from build123d import *

# Parameters (mm, degrees)
F0_R     = 1.25
F1_DEPTH = 18
F2_R     = 6.35
F3_DEPTH = 59.8157


with BuildPart() as f1:
    # F0 (on Top) → F1 (new body)
    with BuildSketch(Plane.XY):
        with BuildLine():
            ThreePointArc((-20.879116, -13.75), (7.17712, -23.947629), (25, 0))
            ThreePointArc((25, 0), (7.17712, 23.947629), (-20.879116, 13.75))
            Line((-20.879116, 13.75), (-20.879116, -13.75))
        make_face()
        Circle(F0_R, mode=Mode.SUBTRACT)
    extrude(amount=F1_DEPTH)

    # F2 (on face) → F3 (cut)
    with BuildSketch(Plane(origin=(-20.879116, 0, 0), x_dir=(0, -1, 0), z_dir=(-1, 0, 0))):
        with Locations((0, 9)):
            Circle(F2_R)
    extrude(amount=-F3_DEPTH, mode=Mode.SUBTRACT)


solid = f1.part
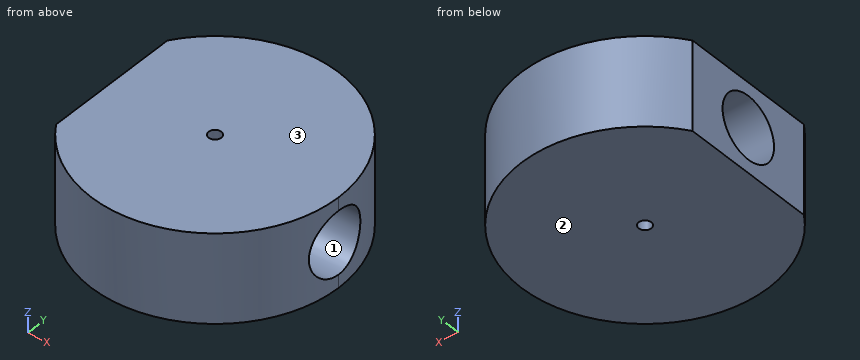
Can you work these out from the model? Positions are in its coordinate system, mm. Face numbers are marked on the shaded views. Give positions to 0.01 mm unless a question says otherwise; leave off trailing zeros. Loops run counter-clockwise (first coordinate to the right, second up) from the corner with the lowest first, then second, coordinate; pieces in that order, holes last. Notation, with made-up numbers: M 75,53.25 L 117,53.25 A27 cw 117,69.25 Z; hole C 72.25,-37 d9. An arc over 180 degrees is marked long. One line per item, written item: value. Start each with the question number.
1) If we section it at C-C, the plane z = 9: Write out the boundary of the cut face in (x, y).
2) If we section it at B-B, the plane y = -3: Write out the boundary of the cut face in (x, z), and give its area (3 significant figures).
3) I'm going to push flat-ended pins straight in: pin 1 (5 mm diameter, centred on x = 17, z = 11.5, fed in from -Y); pin 2 (4 mm diameter, centred on y = 12, z = 3, fed in from +X). Where does each tip first touch, or does it pass through?
4) If we section it at A-A, the plane x = 0: Write out the boundary of the cut face in (y, z), and give its area (3 significant figures).
5) Thinking about a two-plate mould opening in Z: for the marked faces 1, 2 and 3, which applies, +Z half, -Z half, draft (parallel to the pull), parting line (faces both ways), or undercut?
6) If we section it at D-D, the plane z = 16.5: Write out the boundary of the cut face in (x, y), and give its area (3 significant figures).
7) If I drill on line 1 (Y direction, x = 0, z = 16.55); line 2 (Z direction, x = 6, y = 0); line 3 (X direction, y = 0, z = 17.1), over which ranges is the centre line in solid material (lowest first)? Write a range as [from, to].
Completed:
1. outline: M -20.88,-13.75 A25 ccw 24.18,-6.35 L -20.88,-6.35 Z; M -20.88,6.35 L 24.18,6.35 A25 ccw -20.88,13.75 Z
2. outline: M -20.88,0 L 24.82,0 L 24.82,3.4 L -20.88,3.4 Z; M -20.88,14.6 L 24.82,14.6 L 24.82,18 L -20.88,18 Z
2. area: 311 mm^2
3. pin 1: stops at y = -20.37
3. pin 2: stops at x = 22.91
4. outline: M -25,0 L -1.25,0 L -1.25,2.77 A6.35 cw -1.25,15.23 L -1.25,18 L -25,18 Z; M 1.25,0 L 25,0 L 25,18 L 1.25,18 L 1.25,15.23 A6.35 cw 1.25,2.77 Z
4. area: 760 mm^2
5. face 1: undercut
5. face 2: -Z half
5. face 3: +Z half
6. outline: M -20.88,-13.75 A25 ccw long -20.88,13.75 Z; hole C 0,0 d2.5
6. area: 1,880 mm^2
7. line 1: y = [-25, -1.25], [1.25, 25]
7. line 2: z = [0, 2.65], [15.35, 18]
7. line 3: x = [-20.88, -1.25], [1.25, 25]
